Can you work these out from the model? Positions are in its coordinate system, mm. Coordinates: 2 decimals unless noted, no trailing zeros. Order: outer loops, then holes, each group sorted by start corner. A loop starts at its lowest first (then second) coordinate and runs counter-clockwise, first axis right, second up. Notation, with made-up numbers: (51.5, 72) -> (96.5, 72) arc R25 cw to (96.5, 87) -> close; hole circle Ø10 at (41.25, -6.75). An arc over 180 degrees is marked (long way). Answer in a Markdown table with one row per item.
```python
from build123d import *

# Parameters (mm, degrees)
BOSS_EXTRUDE1_DEPTH       = 156.5
M6X1_0_TAPPED_HOLE1_D     = 5
M6X1_0_TAPPED_HOLE1_DEPTH = 17
M6X1_0_TAPPED_HOLE1_TIP   = 1.502151548
M6X1_0_TAPPED_HOLE2_D     = 5
M6X1_0_TAPPED_HOLE2_DEPTH = 17
M6X1_0_TAPPED_HOLE2_TIP   = 1.502151548


with BuildPart() as part:
    # Sketch1 → Boss-Extrude1 (new body)
    with BuildSketch(Plane.XY):
        Polygon((3.452384384, -6.006749709), (6.928190034, -0.013522274), (3.47580565, 5.993227435), (-3.452384384, 6.006749709), (-6.928190034, 0.013522274), (-3.47580565, -5.993227435), align=None)
    extrude(amount=BOSS_EXTRUDE1_DEPTH)

    # M6x1.0 Tapped Hole1
    with Locations(Plane.XY.offset(156.5)):
        with Locations((0, 0)):
            Hole(M6X1_0_TAPPED_HOLE1_D / 2, depth=M6X1_0_TAPPED_HOLE1_DEPTH)
            with Locations((0, 0, -(M6X1_0_TAPPED_HOLE1_DEPTH + M6X1_0_TAPPED_HOLE1_TIP / 2))):  # 118° drill point
                Cone(0, M6X1_0_TAPPED_HOLE1_D / 2, M6X1_0_TAPPED_HOLE1_TIP, mode=Mode.SUBTRACT)

    # M6x1.0 Tapped Hole2
    with Locations(Plane(origin=(0, 0, 0), x_dir=(-1, 0, 0), z_dir=(0, 0, -1))):
        with Locations((0, 0)):
            Hole(M6X1_0_TAPPED_HOLE2_D / 2, depth=M6X1_0_TAPPED_HOLE2_DEPTH)
            with Locations((0, 0, -(M6X1_0_TAPPED_HOLE2_DEPTH + M6X1_0_TAPPED_HOLE2_TIP / 2))):  # 118° drill point
                Cone(0, M6X1_0_TAPPED_HOLE2_D / 2, M6X1_0_TAPPED_HOLE2_TIP, mode=Mode.SUBTRACT)


solid = part.part
```
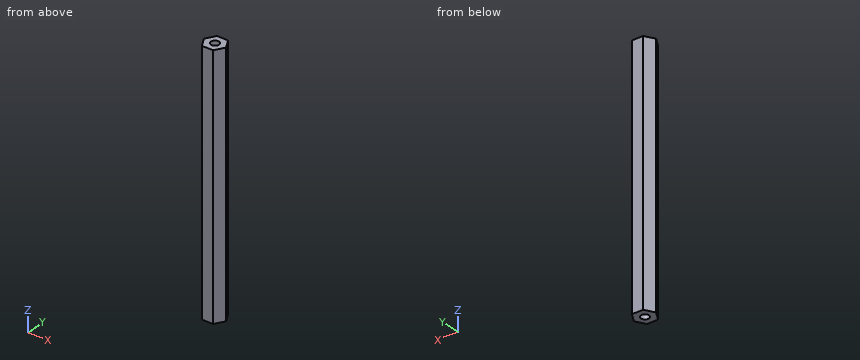
(1) Will these pins go through, and if not, where does the flat tip stop? pin 1 Ø3 at (y, z) = (-2, 134) entering from +X; pin 2 Ø2 at (x, z) = (0, 108.5) entering from +Y; pin 3 Ø2 at (x, y) = (-0.5, 1) entering from -Z.
Response values:
| item | result |
|---|---|
| pin 1 | x = 6.65 |
| pin 2 | y = 6 |
| pin 3 | z = 17.23 |
(2) Suppose I cut it at A-A (z = 144.5). Please give me the cut outline in (x, y).
Response values:
| item | result |
|---|---|
| outline | (-6.93, 0.01) -> (-3.48, -5.99) -> (3.45, -6.01) -> (6.93, -0.01) -> (3.48, 5.99) -> (-3.45, 6.01) -> close; hole circle Ø5 at (0, 0) |
(3) Suppose I cut it at C-C (y = 4.25). Please give me the cut outline in (x, z), and give its area (3 significant figures).
Response values:
| item | result |
|---|---|
| outline | (-4.47, 0) -> (4.48, 0) -> (4.48, 156.5) -> (-4.47, 156.5) -> close |
| area | 1,400 mm2 |
(4) I need wall thicknesses on line 1 (Y direction, x = 0, z = 3.5); line 2 (X direction, y = 0, z = 151.75); line 3 (Y direction, x = -1, z = 52.5). Which ranges of each line are inside material? Lowest first, please. Write a range as [from, to].
Response values:
| item | result |
|---|---|
| line 1 | [-6, -2.5], [2.5, 6] |
| line 2 | [-6.92, -2.5], [2.5, 6.92] |
| line 3 | [-6, 6] |
(5) Suppose I cut it at B-B (z = 76). Please give me the cut outline in (x, y).
Response values:
| item | result |
|---|---|
| outline | (-6.93, 0.01) -> (-3.48, -5.99) -> (3.45, -6.01) -> (6.93, -0.01) -> (3.48, 5.99) -> (-3.45, 6.01) -> close |
